```python
from build123d import *

# Parameters (mm, degrees)
CROQUIS1_W              = 40.5
CROQUIS1_H              = 20.5
SALIENTE_EXTRUIR1_DEPTH = 38.5
SALIENTE_EXTRUIR2_START = -11.5
SALIENTE_EXTRUIR2_DEPTH = 2.5
SALIENTE_EXTRUIR6_DEPTH = 0.6
SIMETR_A2_START         = -11.5
SIMETR_A2_COPY_1_DEPTH  = 2.5
CROQUIS4_W              = 40.5
CROQUIS4_H              = 20.5
CORTAR_EXTRUIR3_DEPTH   = 1.5
CHAFL_N1_SIZE           = 1.5
REDONDEO1_R             = 1
CROQUIS5_R              = 6.75
SALIENTE_EXTRUIR3_DEPTH = 0.3
CROQUIS6_R              = 5.5
SALIENTE_EXTRUIR4_DEPTH = 0.7
CROQUIS7_R              = 2.85
SALIENTE_EXTRUIR5_DEPTH = 4


with BuildPart() as part:
    # Croquis1 → Saliente-Extruir1 (new body)
    with BuildSketch(Plane(origin=(0, 0, 0), x_dir=(1, 0, 0), z_dir=(0, 1, 0))):
        Rectangle(CROQUIS1_W, CROQUIS1_H)
    extrude(amount=SALIENTE_EXTRUIR1_DEPTH)

    # Croquis2 → Saliente-Extruir2 (add)
    with BuildSketch(Plane(origin=(0, 38.5, 0), x_dir=(1, 0, 0), z_dir=(0, 1, 0)).offset(SALIENTE_EXTRUIR2_START)):
        with BuildLine():
            Line((-20.25, 9.5), (-26.1, 9.5))
            ThreePointArc((-26.1, 9.5), (-26.807106781, 9.207106781), (-27.1, 8.5))
            Line((-27.1, 8.5), (-27.1, 6.261088342))
            ThreePointArc((-27.1, 6.261088342), (-21.85, 4.905544171), (-27.1, 3.55))
            Line((-27.1, 3.55), (-27.1, 0))
            Line((-27.1, 0), (-20.25, 0))
            Line((-20.25, 0), (-20.25, 9.5))
        make_face()
    saliente_extruir2 = extrude(amount=SALIENTE_EXTRUIR2_DEPTH)

    # Simetría1: Saliente-Extruir2 across plane
    add(saliente_extruir2.mirror(Plane(origin=(0, 0, 0), x_dir=(1, 0, 0), z_dir=(0, 0, -1))))

    # Croquis8 → Saliente-Extruir6 (add, symmetric)
    with BuildSketch(Plane.XY):
        Polygon((-27.1, 29.5), (-20.25, 30.099297345), (-20.25, 29.5), align=None)
    saliente_extruir6 = extrude(amount=SALIENTE_EXTRUIR6_DEPTH, both=True)

    # Simetría2: Saliente-Extruir2, Saliente-Extruir6 across plane
    add(saliente_extruir2.mirror(Plane(origin=(0, 0, 0), x_dir=(0, 0, 1), z_dir=(1, 0, 0))))
    add(saliente_extruir6.mirror(Plane(origin=(0, 0, 0), x_dir=(0, 0, 1), z_dir=(1, 0, 0))))

    # Simetría2 copy 1 sketch → Simetría2 copy 1 (add)
    with BuildSketch(Plane(origin=(0, 38.5, 0), x_dir=(-1, 0, 0), z_dir=(0, 1, 0)).offset(SIMETR_A2_START)):
        with BuildLine():
            Line((-20.25, 9.5), (-26.1, 9.5))
            ThreePointArc((-26.1, 9.5), (-26.807106781, 9.207106781), (-27.1, 8.5))
            Line((-27.1, 8.5), (-27.1, 6.261088342))
            ThreePointArc((-27.1, 6.261088342), (-21.85, 4.905544171), (-27.1, 3.55))
            Line((-27.1, 3.55), (-27.1, 0))
            Line((-27.1, 0), (-20.25, 0))
            Line((-20.25, 0), (-20.25, 9.5))
        make_face()
    extrude(amount=SIMETR_A2_COPY_1_DEPTH)

    # Croquis4 → Cortar-Extruir3 (cut)
    with BuildSketch(Plane(origin=(0, 38.5, 0), x_dir=(1, 0, 0), z_dir=(0, 1, 0))):
        Rectangle(CROQUIS4_W, CROQUIS4_H)
        with BuildLine():
            Line((-15.25, 9.5), (-15.25, -9.5))
            Line((-15.25, -9.5), (10.25, -9.5))
            ThreePointArc((10.25, -9.5), (19.75, 0), (10.25, 9.5))
            Line((10.25, 9.5), (-15.25, 9.5))
        make_face(mode=Mode.SUBTRACT)
    extrude(amount=-CORTAR_EXTRUIR3_DEPTH, mode=Mode.SUBTRACT)

    # Chaflán1
    chafl_n1_edges = [part.edges().sort_by_distance(p)[0] for p in [
        (-15.25, 38.5, 0),
    ]]
    chamfer(chafl_n1_edges, length=CHAFL_N1_SIZE - 0.0001)  # a hair under: the kernel refuses the full size

    # Redondeo1
    redondeo1_edges = [part.edges().sort_by_distance(p)[0] for p in [
        (-1.75005, 38.5, -9.5),
        (19.75, 38.5, 0),
        (-1.75005, 38.5, 9.5),
    ]]
    fillet(redondeo1_edges, radius=REDONDEO1_R)

    # Croquis5 → Saliente-Extruir3 (add)
    with BuildSketch(Plane(origin=(0, 38.5, 0), x_dir=(1, 0, 0), z_dir=(0, 1, 0))):
        with Locations(Location((10.25, 0, 0), (0, 0, 90))):
            Circle(CROQUIS5_R)
    extrude(amount=SALIENTE_EXTRUIR3_DEPTH)

    # Croquis6 → Saliente-Extruir4 (add)
    with BuildSketch(Plane(origin=(0, 38.8, 0), x_dir=(1, 0, 0), z_dir=(0, 1, 0))):
        with Locations(Location((10.25, 0, 0), (0, 0, 270))):
            Circle(CROQUIS6_R)
    extrude(amount=SALIENTE_EXTRUIR4_DEPTH)

    # Croquis7 → Saliente-Extruir5 (add)
    with BuildSketch(Plane(origin=(0, 39.5, 0), x_dir=(1, 0, 0), z_dir=(0, 1, 0))):
        with Locations(Location((10.25, 0, 0), (0, 0, 270))):
            Circle(CROQUIS7_R)
    extrude(amount=SALIENTE_EXTRUIR5_DEPTH)


solid = part.part
```
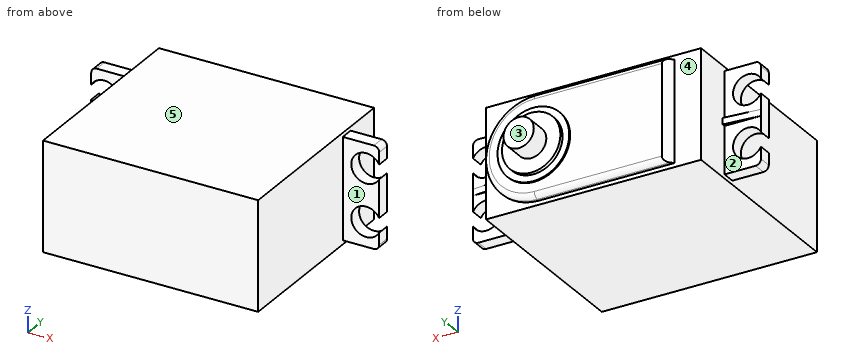
Build history of the part. All positions in model axes, mm. Face numbers are marked on the shaded views. A direction names the side the tool comes from. Round coordinates to 2 decimals unless told otherwise and drop trailing zeros. Order: outer loops, then holes, each group sorted by start corner. A loop starts at its lowest first (then second) coordinate and runs counter-clockwise, first axis right, second up. Notation, with made-up numbers: (80.25, 41) - (96.25, 41) arc R16 cw to (96.25, 64) - close; hole circle Ø3 at (14, 9). An arc over 180 degrees is marked (long way). Use a Markdown table: item, result.
1) Tool access for the marked faces 1, 2, 3, 4 and 5: list every direction of +Z, -Z, +X, -X, +Y, -Y with a clear straight run to the whole face (end or side of a thin tool).
Recorded:
| item | result |
|---|---|
| face 1 | +Z, -Z, +X, -Y |
| face 2 | -Z, -X, +Y |
| face 3 | +Z, -Z, +X, -X, +Y |
| face 4 | +Y |
| face 5 | +Z, +X, -X, +Y, -Y |
2) Saw through at B-B on x = 24.65. Write the cut outline in (y, z).
Recorded:
| item | result |
|---|---|
| outline | (27, -9.5) - (29.5, -9.5) - (29.5, -7.71) - (27, -7.71) - close; (27, -2.11) - (29.5, -2.11) - (29.5, -0.6) - (29.71, -0.6) - (29.71, 0.6) - (29.5, 0.6) - (29.5, 2.11) - (27, 2.11) - close; (27, 7.71) - (29.5, 7.71) - (29.5, 9.5) - (27, 9.5) - close |
3) Saw through at A-A on y = 28. Write the cut outline in (x, z), and give its area (3 significant figures).
Recorded:
| item | result |
|---|---|
| outline | (-27.1, -8.5) arc R1 ccw to (-26.1, -9.5) - (-20.25, -9.5) - (-20.25, -10.25) - (20.25, -10.25) - (20.25, -9.5) - (26.1, -9.5) arc R1 ccw to (27.1, -8.5) - (27.1, -6.26) arc R2.8 cw (long way) to (27.1, -3.55) - (27.1, 3.55) arc R2.8 cw (long way) to (27.1, 6.26) - (27.1, 8.5) arc R1 ccw to (26.1, 9.5) - (20.25, 9.5) - (20.25, 10.25) - (-20.25, 10.25) - (-20.25, 9.5) - (-26.1, 9.5) arc R1 ccw to (-27.1, 8.5) - (-27.1, 6.26) arc R2.8 cw (long way) to (-27.1, 3.55) - (-27.1, -3.55) arc R2.8 cw (long way) to (-27.1, -6.26) - close |
| area | 994 mm² |
4) Saw through at D-D on y = 34. Write the cut outline in (x, z).
Recorded:
| item | result |
|---|---|
| outline | (-20.25, -10.25) - (20.25, -10.25) - (20.25, 10.25) - (-20.25, 10.25) - close |
5) Wall check: L1, parallel to Z at x = -24.65, y = 28.4; L2, parallel to Z at x = -24, y = 29; L3, parallel to X at y = 22, z = -8. Give the ranges that are in metal, low to high.
Recorded:
| item | result |
|---|---|
| L1 | z = -9.5 to -7.71, -2.11 to 2.11, 7.71 to 9.5 |
| L2 | z = -9.5 to -7.63, -2.18 to 2.18, 7.63 to 9.5 |
| L3 | x = -20.25 to 20.25 |
6) Flat gauge pins, fed straight in: pin 1 Ø5.5 at (x, z) = (-25, 4.5) entering from +Y; pin 2 Ø1.5 at (y, z) = (36.5, 3) entering from +X; pin 3 Ø2 at (x, z) = (23, 2) entering from -Y. Where does each tip first touch, or does it go through?
Recorded:
| item | result |
|---|---|
| pin 1 | stops at y = 29.5 |
| pin 2 | stops at x = 20.25 |
| pin 3 | stops at y = 27 |
